```python
from build123d import *

# Parameters (mm, degrees)
F0_W     = 165.1
F0_H     = 114.3
F0_R     = 3.175
F1_DEPTH = 12.7
F2_W     = 165.1
F2_H     = 114.3
F3_DEPTH = 3.175
F4_R     = 5.08


with BuildPart() as f1:
    # F0 (on Top) → F1 (new body)
    with BuildSketch(Plane.XY):
        Rectangle(F0_W, F0_H)
        with Locations((-71.40575, -46.00575)):
            Circle(F0_R, mode=Mode.SUBTRACT)
        with Locations((-61.81725, -46.00575)):
            Circle(F0_R, mode=Mode.SUBTRACT)
        with Locations((-47.171459, -43.434)):
            Circle(F0_R, mode=Mode.SUBTRACT)
        with Locations((-71.40575, -35.78225)):
            Circle(F0_R, mode=Mode.SUBTRACT)
        with Locations((-61.81725, -35.78225)):
            Circle(F0_R, mode=Mode.SUBTRACT)
        with Locations((-32.439459, -43.434)):
            Circle(F0_R, mode=Mode.SUBTRACT)
        with Locations((-12.839662, -41.148)):
            Circle(F0_R, mode=Mode.SUBTRACT)
        with Locations((-71.40575, -25.55875)):
            Circle(F0_R, mode=Mode.SUBTRACT)
        with Locations((-71.40575, -15.33525)):
            Circle(F0_R, mode=Mode.SUBTRACT)
        with Locations((-61.81725, -25.55875)):
            Circle(F0_R, mode=Mode.SUBTRACT)
        with Locations((-47.171459, -26.0604)):
            Circle(F0_R, mode=Mode.SUBTRACT)
        with Locations((-61.81725, -15.33525)):
            Circle(F0_R, mode=Mode.SUBTRACT)
        with Locations((-71.40575, -5.11175)):
            Circle(F0_R, mode=Mode.SUBTRACT)
        with Locations((-47.171459, -8.6868)):
            Circle(F0_R, mode=Mode.SUBTRACT)
        with Locations((-61.81725, -5.11175)):
            Circle(F0_R, mode=Mode.SUBTRACT)
        with Locations((-32.439459, -26.0604)):
            Circle(F0_R, mode=Mode.SUBTRACT)
        with Locations((-12.839662, -20.574)):
            Circle(F0_R, mode=Mode.SUBTRACT)
        with Locations((-32.439459, -8.6868)):
            Circle(F0_R, mode=Mode.SUBTRACT)
        with Locations((6.464338, -41.148)):
            Circle(F0_R, mode=Mode.SUBTRACT)
        with Locations((30.402271, -38.1)):
            Circle(F0_R, mode=Mode.SUBTRACT)
        with Locations((60.325, -34.925)):
            Circle(F0_R, mode=Mode.SUBTRACT)
        with Locations((6.464338, -20.574)):
            Circle(F0_R, mode=Mode.SUBTRACT)
        with Locations((30.402271, -12.7)):
            Circle(F0_R, mode=Mode.SUBTRACT)
        with Locations((-71.40575, 5.11175)):
            Circle(F0_R, mode=Mode.SUBTRACT)
        with Locations((-61.81725, 5.11175)):
            Circle(F0_R, mode=Mode.SUBTRACT)
        with Locations((-47.171459, 8.6868)):
            Circle(F0_R, mode=Mode.SUBTRACT)
        with Locations((-71.40575, 15.33525)):
            Circle(F0_R, mode=Mode.SUBTRACT)
        with Locations((-71.40575, 25.55875)):
            Circle(F0_R, mode=Mode.SUBTRACT)
        with Locations((-61.81725, 15.33525)):
            Circle(F0_R, mode=Mode.SUBTRACT)
        with Locations((-61.81725, 25.55875)):
            Circle(F0_R, mode=Mode.SUBTRACT)
        with Locations((-47.171459, 26.0604)):
            Circle(F0_R, mode=Mode.SUBTRACT)
        with Locations((-32.439459, 8.6868)):
            Circle(F0_R, mode=Mode.SUBTRACT)
        with Locations((-12.839662, 0)):
            Circle(F0_R, mode=Mode.SUBTRACT)
        with Locations((-32.439459, 26.0604)):
            Circle(F0_R, mode=Mode.SUBTRACT)
        with Locations((-12.839662, 20.574)):
            Circle(F0_R, mode=Mode.SUBTRACT)
        with Locations((-71.40575, 35.78225)):
            Circle(F0_R, mode=Mode.SUBTRACT)
        with Locations((-61.81725, 35.78225)):
            Circle(F0_R, mode=Mode.SUBTRACT)
        with Locations((-71.40575, 46.00575)):
            Circle(F0_R, mode=Mode.SUBTRACT)
        with Locations((-61.81725, 46.00575)):
            Circle(F0_R, mode=Mode.SUBTRACT)
        with Locations((-47.171459, 43.434)):
            Circle(F0_R, mode=Mode.SUBTRACT)
        with Locations((-12.839662, 41.148)):
            Circle(F0_R, mode=Mode.SUBTRACT)
        with Locations((-32.439459, 43.434)):
            Circle(F0_R, mode=Mode.SUBTRACT)
        with Locations((6.464338, 0)):
            Circle(F0_R, mode=Mode.SUBTRACT)
        with Locations((30.402271, 12.7)):
            Circle(F0_R, mode=Mode.SUBTRACT)
        with Locations((6.464338, 20.574)):
            Circle(F0_R, mode=Mode.SUBTRACT)
        with Locations((60.325, 0)):
            Circle(F0_R, mode=Mode.SUBTRACT)
        with Locations((6.464338, 41.148)):
            Circle(F0_R, mode=Mode.SUBTRACT)
        with Locations((30.402271, 38.1)):
            Circle(F0_R, mode=Mode.SUBTRACT)
        with Locations((60.325, 34.925)):
            Circle(F0_R, mode=Mode.SUBTRACT)
    extrude(amount=-F1_DEPTH)

    # F2 (on face) → F3 (join)
    with BuildSketch(Plane(origin=(0, 0, -12.7), x_dir=(1, 0, 0), z_dir=(0, 0, -1))):
        Rectangle(F2_W, F2_H)
    extrude(amount=F3_DEPTH)

    # F4
    f4_edges = [f1.edges().sort_by_distance(p)[0] for p in [
        (-82.55, -57.15, -7.9375),
        (-82.55, 57.15, -7.9375),
        (82.55, -57.15, -7.9375),
        (82.55, 57.15, -7.9375),
    ]]
    fillet(f4_edges, radius=F4_R)


solid = f1.part
```
For this review, take the finished solid that the model builds, in its own axes (mm). Give positions to 0.01 mm unless a question says otherwise; leave off trailing zeros. Order: outer loops, then holes, each group sorted by start corner. A loop starts at its lowest first (then second) coordinate and runs counter-clockwise, first axis right, second up.
1) The part is to be moulded in two halves that separate along Y. For faces 1 (the face through (-15.36, 18.64, -6.26)), 2 (the face through (-1, 1, 0)), say which applies: released by +Y, released by -Y, zero draft, split by the parting line, or undercut.
2) Take a section at A-A (y = 0). Give the boundary of the cut face in (x, z) (3 decimals).
3) Wall thickness on line 1 (Y direction, x = 60, z = -6.75); line 2 (Y direction, x = -14.5, z = -1.75); line 3 (X direction, y = 45.5, z = -7.25): over which ranges is each line inside the solid? List them lowest first.
4) Take a section at B-B (x = -31). Give the boundary of the cut face in (y, z) (3 decimals).
5) Take a section at C-C (z = -11). State how many separate pieces and enclosed holes the cut face has, then the cut area to 3 significant figures.
6) Insertion check: pin 1 (5.5 mm diameter, centred on x = 30.4, y = -12.7, fed in from +Z). The pin has a flat end and moves straight along its axis. Give the tip position at first contact, or say it passes through.
Derived:
1. face 1: undercut
1. face 2: zero draft
2. outline: (-82.55, -15.875) - (82.55, -15.875) - (82.55, 0) - (63.5, 0) - (63.5, -12.7) - (57.15, -12.7) - (57.15, 0) - (9.639, 0) - (9.639, -12.7) - (3.289, -12.7) - (3.289, 0) - (-9.665, 0) - (-9.665, -12.7) - (-16.015, -12.7) - (-16.015, 0) - (-82.55, 0) - close
3. line 1: y = -57.15 to -38.08, -31.77 to -3.16, 3.16 to 31.77, 38.08 to 57.15
3. line 2: y = -57.15 to -43.85, -38.44 to -23.28, -17.87 to -2.71, 2.71 to 17.87, 23.28 to 38.44, 43.85 to 57.15
3. line 3: x = -82.55 to -74.54, -68.27 to -64.95, -58.68 to -49.58, -44.76 to -34.85, -30.03 to 82.55
4. outline: (-57.15, -15.875) - (57.15, -15.875) - (57.15, 0) - (46.264, 0) - (46.264, -12.7) - (40.604, -12.7) - (40.604, 0) - (28.89, 0) - (28.89, -12.7) - (23.23, -12.7) - (23.23, 0) - (11.517, 0) - (11.517, -12.7) - (5.857, -12.7) - (5.857, 0) - (-5.857, 0) - (-5.857, -12.7) - (-11.517, -12.7) - (-11.517, 0) - (-23.23, 0) - (-23.23, -12.7) - (-28.89, -12.7) - (-28.89, 0) - (-40.604, 0) - (-40.604, -12.7) - (-46.264, -12.7) - (-46.264, 0) - (-57.15, 0) - close
5. separate pieces: 1
5. enclosed holes: 49
5. area: 17,300 mm2
6. pin 1: stops at z = -12.7
